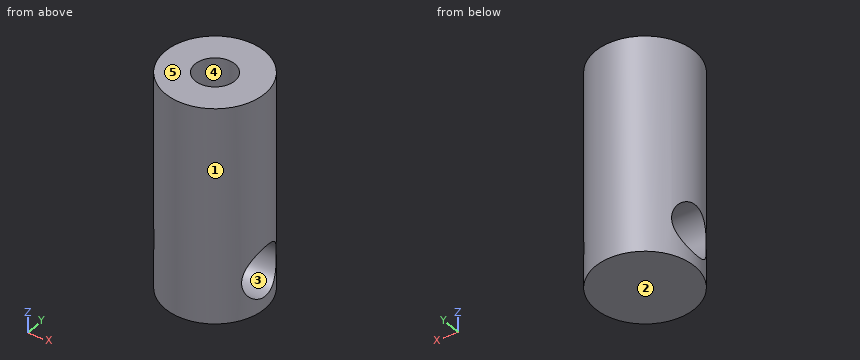
```python
from build123d import *

# Parameters (mm, degrees)
SKETCH1_R               = 6.35
BOSS_EXTRUDE1_DEPTH     = 27.6225
CUT_EXTRUDE2_DEPTH      = 30.045610791
CUT_EXTRUDE2_DEPTH_BACK = 30.045610791
SKETCH3_R               = 3.175
SKETCH2_2_R             = 2.54
CUT_EXTRUDE3_DEPTH      = 12.7


with BuildPart() as part:
    # Sketch1 → Boss-Extrude1 (new body)
    with BuildSketch(Plane.XY):
        Circle(SKETCH1_R)
    extrude(amount=BOSS_EXTRUDE1_DEPTH)

    # Sketch3 → Cut-Extrude2 (cut, two sides: drawn at the far end of the back side and taken through both)
    with BuildSketch(Plane(origin=(0, 0, 0), x_dir=(0, 0, -1), z_dir=(1, 0, 0)).offset(-CUT_EXTRUDE2_DEPTH_BACK)):
        with Locations((-4.7625, 0)):
            Circle(SKETCH3_R)
    extrude(amount=CUT_EXTRUDE2_DEPTH + CUT_EXTRUDE2_DEPTH_BACK, mode=Mode.SUBTRACT)

    # Sketch2<2> → Cut-Extrude3 (cut)
    with BuildSketch(Plane.XY.offset(27.6225)):
        Circle(SKETCH2_2_R)
    extrude(amount=-CUT_EXTRUDE3_DEPTH, mode=Mode.SUBTRACT)


solid = part.part
```
For this review, take the finished solid that the model builds, in its own axes (mm). Face numbers are marked on the shaded views. A direction names the side the tool comes from. Coordinates: 2 decimals unless noted, no trailing zeros. Write each loop counter-clockwise with the first axis right and the second up, starting at its lowest first coordinate (ties: lowest second). Pieces come first, ordered by that corner, then holes. Notation, with made-up numbers: (-24.5, 9.25) - (-19.5, 9.25) arc R16 cw to (-19.5, 33.25) - close; hole circle Ø11 at (7, 54). An arc over 180 degrees is marked (long way). Put each result on its own line as item: value.
1. Machinability: for the marked faces 4 and 5, which of the approach directions +Z, -Z, +X, -X, +Y, -Y give a long, thin tool a straight path to every point of the face, cutting with its end or side? Answer none if there is none.
Values found:
face 4: +Z
face 5: +Z, +X, -X, +Y, -Y
2. Add section C-C, the plane z = 25.75. Give the boundary of the cut face in (x, y).
Values found:
outline: circle Ø12.7 at (0, 0); hole circle Ø5.08 at (0, 0)
3. Wall thickness on probe 1 along Y at (x, z) = (0, 23); probe 2 along Z at (x, y) = (-2.25, 0); probe 3 along Y at (x, z) = (1, 20.5): over which ranges is each line inside the solid? List them lowest first.
Values found:
probe 1: -6.35 to -2.54, 2.54 to 6.35
probe 2: 0 to 1.59, 7.94 to 14.92
probe 3: -6.27 to -2.33, 2.33 to 6.27
4. Mouldability with a two-part tool opening along Y and no side actions: class the marked faces 1, 2 and 3 as released by +Y, released by -Y, zero draft, split by the parting line, or undercut.
Values found:
face 1: split by the parting line
face 2: zero draft
face 3: undercut
5. Add section A-A, the plane y = 0. Give the boundary of the cut face in (x, z).
Values found:
outline: (-6.35, 0) - (6.35, 0) - (6.35, 1.59) - (-6.35, 1.59) - close; (-6.35, 7.94) - (6.35, 7.94) - (6.35, 27.62) - (2.54, 27.62) - (2.54, 14.92) - (-2.54, 14.92) - (-2.54, 27.62) - (-6.35, 27.62) - close
6. For pin 1 (2 mm diameter, centred on y = -4, z = 8, fed in from -X); pin 2 (5 mm diameter, centred on y = 4.5, z = 5, fed in from -X); pin 3 (2 mm diameter, centred on x = -3.5, z = 15.5, fed in from -Y), all flat-tipped, find the tip position at first contact; note any pin that passes through.
Values found:
pin 1: x = -5.6
pin 2: x = -5.8
pin 3: y = -5.84
